Part print with two shaded views. Sizes in mm from the minimum x, y, z corner. A direction names the side the tool comes from. Round coordinates to 2 decimals unless told otherwise and drop trailing zeros. Loops run counter-clockwise (first coordinate to the right, second up) from the corner with the lowest first, then second, coordinate; pieces in that order, holes last.
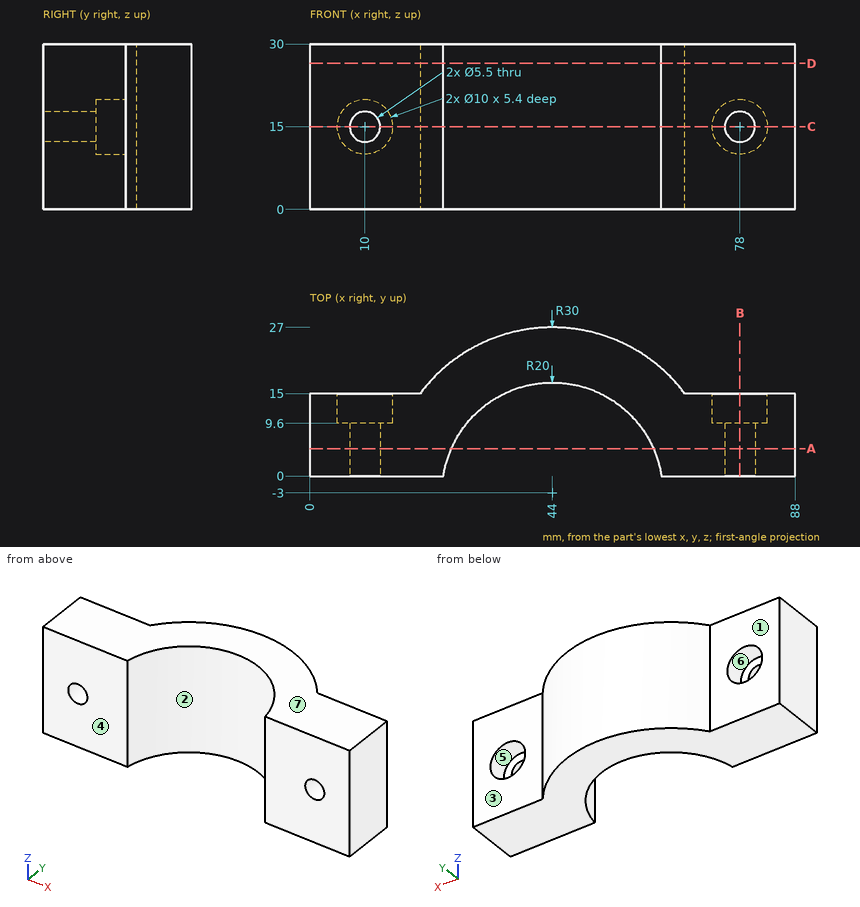
Item 1: Flat gauge pins, fed straight in: P1, Ø6, axis at x = 52, z = 25, coming from the +Y side; P2, Ø16, axis at x = 78, z = 15, coming from the +Y side; P3, Ø1, axis at x = 58, z = 26, coming from the +Y side. Where does each tip first touch, or does it go through?
Verdict:
P1: stops at y = 26.58
P2: stops at y = 15
P3: stops at y = 23.79
Item 2: 3-axis set-ups, long thin cutter, end or side, ignore diameter. For the marked faces 1, 2 and 3: which of +Z, -Z, +X, -X, +Y, -Y reach the whole face in a straight line?
Verdict:
face 1: +Z, -Z, -X, +Y
face 2: +Z, -Z, -Y
face 3: +Z, -Z, +X, +Y
Item 3: Cut at C-C (z = 15). List the corners of the cut face in (x, y), plus the area to 3 significant figures.
Verdict:
outline: (0, 0) - (7.25, 0) - (7.25, 9.6) - (5, 9.6) - (5, 15) - (0, 15) - close; (12.75, 0) - (24.23, 0) arc R20 cw to (63.77, 0) - (75.25, 0) - (75.25, 9.6) - (73, 9.6) - (73, 15) - (68, 15) arc R30 ccw to (20, 15) - (15, 15) - (15, 9.6) - (12.75, 9.6) - close; (80.75, 0) - (88, 0) - (88, 15) - (83, 15) - (83, 9.6) - (80.75, 9.6) - close
area: 1,000 mm2
Item 4: Cut at D-D (z = 26.5). List the corners of the cut face in (x, y), plus the area to 3 significant figures.
Verdict:
outline: (0, 0) - (24.23, 0) arc R20 cw to (63.77, 0) - (88, 0) - (88, 15) - (68, 15) arc R30 ccw to (20, 15) - (0, 15) - close
area: 1,210 mm2
Item 5: Cut at B-B (x = 78). List the corners of the cut face in (y, z), plus the area to 3 significant figures.
Verdict:
outline: (0, 0) - (15, 0) - (15, 10) - (9.6, 10) - (9.6, 12.25) - (0, 12.25) - close; (0, 17.75) - (9.6, 17.75) - (9.6, 20) - (15, 20) - (15, 30) - (0, 30) - close
area: 343 mm2
Item 6: Wall check: L1, parallel to X at y = 12.3, z = 15; L2, parallel to X at y = 12.8, z = 15; L3, parallel to Y at x = 76.5, z = 20.5. Give the ranges that are in metal, low to high.
Verdict:
L1: x = 0 to 5, 15 to 31.12, 56.88 to 73, 83 to 88
L2: x = 0 to 5, 15 to 31.74, 56.26 to 73, 83 to 88
L3: y = 0 to 15
Item 7: Cut at A-A (y = 5). List the corners of the cut face in (x, z), plus the area to 3 significant figures.
Verdict:
outline: (0, 0) - (25.67, 0) - (25.67, 30) - (0, 30) - close; (62.33, 0) - (88, 0) - (88, 30) - (62.33, 30) - close; hole circle Ø5.5 at (10, 15); hole circle Ø5.5 at (78, 15)
area: 1,490 mm2
Item 8: Mould opens along Z. For the marked faces 4, 5, 6 and 7 say: released by +Z, released by -Z, zero draft, split by the parting line, or undercut.
Verdict:
face 4: zero draft
face 5: undercut
face 6: undercut
face 7: released by +Z
